For this review, take the finished solid that the model builds, in its own axes (mm). Round coordinates to 2 decimals unless told otherwise and drop trailing zeros. Order: outer loops, then holes, each group sorted by start corner. A loop starts at its lowest first (then second) coordinate and runs counter-clockwise, first axis right, second up. Notation, with made-up numbers: M 31.5,31.25 L 69.5,31.25 A21 cw 69.5,59.25 Z; hole C 83,54 d2. An arc over 180 degrees is marked long. Answer in a Markdown table with one row per item. Add a question column.
Autodesk Inventor part; units mm, degrees
ref_plane "YZ Plane" through (0, 0, 0) normal (1, 0, 0) x (0, 1, 0)
ref_plane "XZ Plane" through (0, 0, 0) normal (0, 1, 0) x (-1, 0, 0)
ref_plane "XY Plane" through (0, 0, 0) normal (0, 0, 1) x (1, 0, 0)
sketch "Sketch1" plane through (0, 0, 0) normal (0, 1, 0) x (-1, 0, 0)
  line L0 (0, 0) -> (0, -382.775) construction
  line L1 (-5, 0) -> (-5, -382.775)
  line L2 (5, -382.775) -> (5, 0)
  arc A0 (5, 0) -> (-5, 0) centre (0, 0) ccw
  arc A1 (-5, -382.775) -> (5, -382.775) centre (0, -382.775) ccw
  circle A2 centre (0, 0) radius 1.5
  circle A3 centre (0, -382.775) radius 1.5
  arc A4 (5, -382.775) -> (5, 0) centre (-346.2418, -191.3875) ccw
  arc A5 (-5, -382.775) -> (-5, 0) centre (-356.2418, -191.3875) ccw
  point P0 (0, -191.3875)
  dimension "d0" = 382.775
  dimension "d1" = 10
  dimension "d2" = 3
  dimension "d3" = 3
  dimension "d12" = 400
  dimension "d13" = 400
extrude "Extrusion1" add sketch "Sketch1" along normal blind 8 contours A0 L2 A5 | A5 L2 A1 | A4 L2 A5
fillet "Fillet1" radius 2 4 edges at (5, 4, -382.775) (-5, 4, -382.775) (-5, 4, 0) (5, 4, 0)
sketch "Sketch2" plane through (0, 0, 0) normal (0, -1, 0) x (1, 0, 0)
  arc A0 (-4.9846, -383.1668) -> (4.9441, -383.5202) centre (0, -382.775) ccw
  arc A1 (4.9441, 0.7452) -> (-4.9846, 0.3918) centre (0, 0) ccw
  circle A2 centre (0, -382.775) radius 1.5
  circle A3 centre (0, 0) radius 1.5
  arc A4 (-5.2212, -0.4065) -> (-5.2212, -382.3685) centre (346.2418, -191.3875) ccw
  arc A5 (4.7241, -0.5073) -> (4.7241, -382.2677) centre (356.2418, -191.3875) ccw
  arc A6 (4.7241, -0.5073) -> (4.9441, 0.7452) centre (2.9665, 0.4471) ccw
  arc A7 (-5.2212, -0.4065) -> (-4.9846, 0.3918) centre (-6.9785, 0.5485) ccw
  arc A8 (-4.9846, -383.1668) -> (-5.2212, -382.3685) centre (-6.9785, -383.3235) ccw
  arc A9 (4.9441, -383.5202) -> (4.7241, -382.2677) centre (2.9665, -383.2221) ccw
sketch "Sketch3" plane through (0, 8, 0) normal (0, 1, 0) x (1, 0, 0)
  line L0 (-111.727, 425.5197) -> (93.4733, 425.5197)
  line L1 (93.4733, 425.5197) -> (93.4733, -68.38)
  line L2 (93.4733, -68.38) -> (-111.727, -68.38)
  line L3 (-111.727, -68.38) -> (-111.727, 425.5197)
  line L4 (-64.7929, 400.3549) -> (33.9871, 400.3549)
  line L5 (33.9871, 400.3549) -> (33.9871, 210)
  line L6 (33.9871, 210) -> (-64.7929, 210)
  line L7 (-64.7929, 210) -> (-64.7929, 400.3549)
  line L8 (-64.7929, 210) -> (33.9871, 210)
  line L9 (33.9871, 210) -> (33.9871, 30)
  line L10 (33.9871, 30) -> (-64.7929, 30)
  line L11 (-64.7929, 30) -> (-64.7929, 210)
  point P0 (0, 0)
  dimension "d15" = 30
  dimension "d16" = 180
  dimension "d17" = 190.3549
extrude "Extrusion2" cut sketch "Sketch3" along normal mid plane 20 contours L0 L1 L2 L3 | L4 L5 L6 L7
sketch "Sketch4" plane through (0, 8, 0) normal (0, 1, 0) x (1, 0, 0)
  line L0 (-43.3249, 210) -> (-53.3249, 210)
  arc A0 (-43.3249, 210) -> (-9.7555, 30) centre (356.2418, 191.3875) ccw
  arc A1 (-53.3249, 210) -> (-19.7555, 30) centre (346.2418, 191.3875) ccw
  line L1 (-19.7555, 30) -> (-9.7555, 30)
  point P0 (0, 0)
properties part number "Part_13_p2"
1. The part is to be moulded in two halves that separate along Z. For faces 1 (the flat face through (-15, 4, -30)), 2 (the flat face through (-48, 4, -210)), 3 (the cylindrical face through (-36.74, 3.94, -116.78)), say which applies: pulls with the +Z half, pulls with the -Z half, needs draft (parallel to the pull), parting line crosses it, or undercut.
2. Consider section B-B on z = -93.5. Write out the cut boundary in (x, y).
3. Clearance check with flat-ended pins moving along their axes: pin 1 Ø4 at (y, z) = (5.5, -131) entering from +X; pin 2 Ø2 at (y, z) = (1.5, -159) entering from +X; pin 3 Ø1.5 at (y, z) = (4.5, -57) entering from +X. State where each tip first meets the part, or that it passes through.
4. Consider section A-A on y = 2.75. Write out the cut boundary in (x, z), plus the area to 3 significant figures.
5. To check wall thickness, follow probe 1 along X at (y, z) = (4.5, -188); probe 2 along X at (y, z) = (6.25, -74.5); probe 3 along Z at (x, y) = (-13, 4.75). State the ranges of each line that lie inside material, in increasing order. Write a range as [from, to].
Solved:
| question | item | result |
|---|---|---|
| 1 | face 1 | pulls with the +Z half |
| 1 | face 2 | pulls with the -Z half |
| 1 | face 3 | undercut |
| 2 | outline | M -41.6,0 L -31.6,0 L -31.6,8 L -41.6,8 Z |
| 3 | pin 1 | stops at x = -38.86 |
| 3 | pin 2 | stops at x = -42.36 |
| 3 | pin 3 | stops at x = -20.24 |
| 4 | outline | M -53.32,-210 L -43.32,-210 A400 cw -9.76,-30 L -19.76,-30 A400 ccw Z |
| 4 | area | 1,800 mm^2 |
| 5 | probe 1 | x = [-53.74, -43.74] |
| 5 | probe 2 | x = [-36.3, -26.3] |
| 5 | probe 3 | z = [-37.57, -30] |
